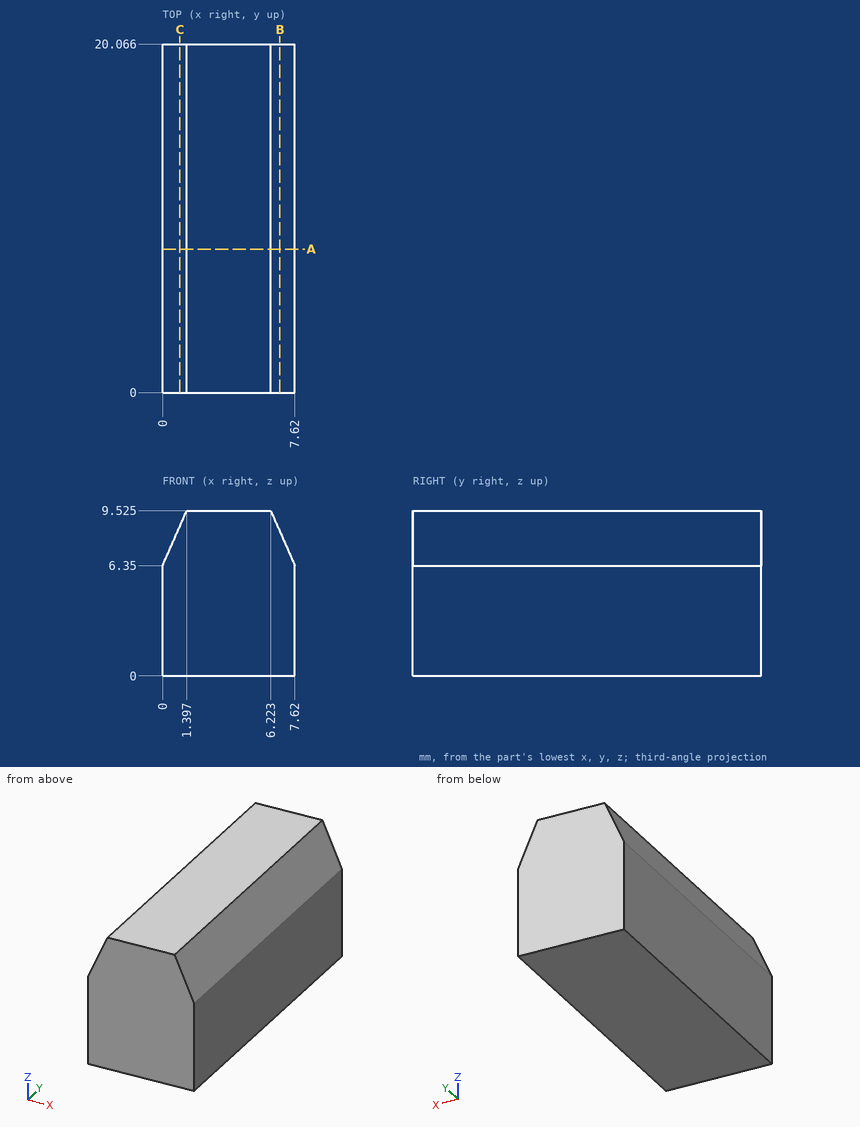
Drawing for the job (mm, zero at the part's lowest x, y, z). Round coordinates to 2 decimals unless told otherwise and drop trailing zeros. Loops run counter-clockwise (first coordinate to the right, second up) from the corner with the lowest first, then second, coordinate; pieces in that order, holes last.
1. Wall check: probe 1 along X at (y, z) = (1.25, 8); probe 2 along X at (y, z) = (4.5, 9.25); probe 3 along Z at (x, y) = (0.75, 11.75). Give the ranges that are in metal, low to high.
Check values:
probe 1: x = 0.73 to 6.89
probe 2: x = 1.28 to 6.34
probe 3: z = 0 to 8.05
2. Band-saw the part on B-B, the plane x = 6.75. List the corners of the cut face in (y, z).
Check values:
outline: (0, 0) - (20.07, 0) - (20.07, 8.33) - (0, 8.33) - close
3. Band-saw the part on C-C, the plane x = 1. List the corners of the cut face in (y, z), and give its area (3 significant figures).
Check values:
outline: (0, 0) - (20.07, 0) - (20.07, 8.62) - (0, 8.62) - close
area: 173 mm2
4. Drop flat-ended pins along their axis: P1, Ø3, axis at x = 1.5, y = 14.5, coming from the -Z side; P2, Ø2, axis at y = 8.5, z = 8, coming from the -X side. Give the stop position or say it passes through.
Check values:
P1: stops at z = 0
P2: stops at x = 0.29
5. Band-saw the part on A-A, the plane y = 8.25. List the corners of the cut face in (x, z) (3 decimals), and give its area (3 significant figures).
Check values:
outline: (0, 0) - (7.62, 0) - (7.62, 6.35) - (6.223, 9.525) - (1.397, 9.525) - (0, 6.35) - close
area: 68.1 mm2
